Read the model definition and answer for the solid it produces. Units are mm, in the model's axes. A direction names the side the tool comes from. Coordinates: 2 decimals unless noted, no trailing zeros. Order: outer loops, then holes, each group sorted by start corner. A loop starts at its lowest first (then second) coordinate and runs counter-clockwise, first axis right, second up. Notation, with made-up numbers: M 6,49 L 59,49 A9 ccw 59,59 Z; hole C 63,57 d3. An arc over 180 degrees is marked long. Put each result on its own line as item: value.
from build123d import *

# Parameters (mm, degrees)
F0_R     = 1.5
F0_R_2   = 11
F1_DEPTH = 15
F2_W     = 10
F2_H     = 10
F3_DEPTH = 20
F4_W     = 15
F4_H     = 15
F4_W_2   = 10
F4_H_2   = 10
F5_DEPTH = 20
F6_F1_R  = 5
F6_F2_R  = 5
F6_F3_R  = 5
F6_F4_R  = 5
F6_F5_R  = 5
F6_F6_R  = 5
F6_F7_R  = 5
F6_F8_R  = 5
F6_F9_R  = 5
F6_F10_R = 5
F6_F11_R = 5
F6_F12_R = 5
F6_F13_R = 5
F7_R     = 4
F8_DEPTH = 7.5
F9_R     = 5


with BuildPart() as f1:
    # F0 (on Top) → F1 (new body)
    with BuildSketch(Plane.XY):
        with BuildLine():
            Line((-45, -32.5), (-45, -45))
            Line((-45, -45), (-30, -45))
            Line((-30, -45), (-30, -60))
            Line((-30, -60), (-15, -60))
            Line((-15, -60), (-15, -45))
            Line((-15, -45), (0, -45))
            Line((0, -45), (0, -32.5))
            ThreePointArc((0, -32.5), (10, -22.5), (0, -12.5))
            Line((0, -12.5), (0, 0))
            Line((0, 0), (-15, 0))
            Line((-15, 0), (-15, 15))
            Line((-15, 15), (-30, 15))
            Line((-30, 15), (-30, 0))
            Line((-30, 0), (-45, 0))
            Line((-45, 0), (-45, -12.5))
            ThreePointArc((-45, -12.5), (-55, -22.5), (-45, -32.5))
        make_face()
        with Locations((-38, -38)):
            Circle(F0_R, mode=Mode.SUBTRACT)
        with Locations((-7, -38)):
            Circle(F0_R, mode=Mode.SUBTRACT)
        with Locations((-38, -7)):
            Circle(F0_R, mode=Mode.SUBTRACT)
        with Locations((-22.5, -22.5)):
            Circle(F0_R_2, mode=Mode.SUBTRACT)
        with Locations((-7, -7)):
            Circle(F0_R, mode=Mode.SUBTRACT)
    extrude(amount=F1_DEPTH)

    # F2 (on face) → F3 (cut)
    with BuildSketch(Plane.XZ.offset(60)):
        with Locations((-22.5, 7.5)):
            Rectangle(F2_W, F2_H)
    extrude(amount=-F3_DEPTH, mode=Mode.SUBTRACT)

    # F4 (on face) → F5 (join)
    with BuildSketch(Plane.XY.offset(15)):
        with Locations((-22.5, 7.5)):
            Rectangle(F4_W, F4_H)
        with Locations((-22.5, 7.5)):
            Rectangle(F4_W_2, F4_H_2, mode=Mode.SUBTRACT)
    extrude(amount=F5_DEPTH)

    # F6: fillet of radius 5 on 13 edges, made by hand

    # F6_f1
    f6_f1_edges = [f1.edges().sort_by_distance(p)[0] for p in [
        (-15, 0, 7.5),
    ]]
    fillet(f6_f1_edges, radius=F6_F1_R)

    # F6_f2
    f6_f2_edges = [f1.edges().sort_by_distance(p)[0] for p in [
        (-22.5, 0, 15),
    ]]
    fillet(f6_f2_edges, radius=F6_F2_R)

    # F6_f3
    f6_f3_edges = [f1.edges().sort_by_distance(p)[0] for p in [
        (0, -12.5, 7.5),
    ]]
    fillet(f6_f3_edges, radius=F6_F3_R)

    # F6_f4
    f6_f4_edges = [f1.edges().sort_by_distance(p)[0] for p in [
        (0, 0, 7.5),
    ]]
    fillet(f6_f4_edges, radius=F6_F4_R)

    # F6_f5
    f6_f5_edges = [f1.edges().sort_by_distance(p)[0] for p in [
        (0, -32.5, 7.5),
    ]]
    fillet(f6_f5_edges, radius=F6_F5_R)

    # F6_f6
    f6_f6_edges = [f1.edges().sort_by_distance(p)[0] for p in [
        (0, -45, 7.5),
    ]]
    fillet(f6_f6_edges, radius=F6_F6_R)

    # F6_f7
    f6_f7_edges = [f1.edges().sort_by_distance(p)[0] for p in [
        (-15, -45, 7.5),
    ]]
    fillet(f6_f7_edges, radius=F6_F7_R)

    # F6_f8
    f6_f8_edges = [f1.edges().sort_by_distance(p)[0] for p in [
        (-30, -45, 7.5),
    ]]
    fillet(f6_f8_edges, radius=F6_F8_R)

    # F6_f9
    f6_f9_edges = [f1.edges().sort_by_distance(p)[0] for p in [
        (-45, -45, 7.5),
    ]]
    fillet(f6_f9_edges, radius=F6_F9_R)

    # F6_f10
    f6_f10_edges = [f1.edges().sort_by_distance(p)[0] for p in [
        (-45, -32.5, 7.5),
    ]]
    fillet(f6_f10_edges, radius=F6_F10_R)

    # F6_f11
    f6_f11_edges = [f1.edges().sort_by_distance(p)[0] for p in [
        (-45, -12.5, 7.5),
    ]]
    fillet(f6_f11_edges, radius=F6_F11_R)

    # F6_f12
    f6_f12_edges = [f1.edges().sort_by_distance(p)[0] for p in [
        (-45, 0, 7.5),
    ]]
    fillet(f6_f12_edges, radius=F6_F12_R)

    # F6_f13
    f6_f13_edges = [f1.edges().sort_by_distance(p)[0] for p in [
        (-30, 0, 7.5),
    ]]
    fillet(f6_f13_edges, radius=F6_F13_R)

    # F7 (on face) → F8 (cut)
    with BuildSketch(Plane.XY.offset(15)):
        with Locations((-45, -22.5)):
            Circle(F7_R)
        with Locations((0, -22.5)):
            Circle(F7_R)
    extrude(amount=-F8_DEPTH, mode=Mode.SUBTRACT)

    # F9
    f9_edges = [f1.edges().sort_by_distance(p)[0] for p in [
        (-15, 0, 15),
        (-30, 0, 15),
    ]]
    fillet(f9_edges, radius=F9_R)


solid = f1.part
Q1. Consider line 1 along Y through (x, z) = (-38, 11); line 2 along Y through (x, z) = (-22.5, 25.5); line 3 along Y through (x, z) = (-22.5, 11.75). Determine where each line is inside the solid, lowest interval first.
Answers below:
line 1: y = -45 to -39.5, -36.5 to -8.5, -5.5 to 0
line 2: y = 0 to 2.5, 12.5 to 15
line 3: y = -40 to -33.5, -11.5 to 15
Q2. Find section A-A on x = -38. Write down the section's boundary in (y, z).
Answers below:
outline: M -45,0 L -39.5,0 L -39.5,15 L -45,15 Z; M -36.5,0 L -8.5,0 L -8.5,15 L -36.5,15 Z; M -5.5,0 L 0,0 L 0,15 L -5.5,15 Z
Q3. Given pin 1 (1.7 mm diameter, centred on y = -38.5, z = 6.5, fed in from +X); pin 2 (5 mm diameter, centred on y = 7.5, z = 21.5, fed in from -X); pin 3 (5 mm diameter, centred on x = -45, y = -22.5, fed in from +Z), each flat-ended and moving along its own axis, determine where each tip first touches the part or whether it passes through.
Answers below:
pin 1: stops at x = 0
pin 2: stops at x = -30
pin 3: stops at z = 7.5
Q4. For a pull along Y with two mould halves and no side action, classify faces 1 (the face through (-45.943, -11.28, 7.605)), 2 (the face through (-45, -38, 7)), 3 (the face through (-17.5, 7, 25)) as +Y half, -Y half, draft (parallel to the pull), parting line (faces both ways), or undercut.
Answers below:
face 1: +Y half
face 2: draft
face 3: undercut
Q5. Find section C-C on z = 23.5. Write down the section's boundary in (x, y).
Answers below:
outline: M -30,0 L -15,0 L -15,15 L -30,15 Z; hole M -27.5,2.5 L -17.5,2.5 L -17.5,12.5 L -27.5,12.5 Z
Q6. A tool of negligible diameter and unlimited length cuts with its end or side. For faces 4 (the face through (0, -7, 7)), 5 (the face through (-23, 2.5, 25)), 6 (the face through (-15, -55, 7)), from which of +Z, -Z, +X, -X, +Y, -Y can it reach the whole face along a straight path? Write none if from no direction.
Answers below:
face 4: +Z, -Z, +X, +Y
face 5: +Z
face 6: +Z, -Z, +X, -Y
Q7. Find section B-B on y = -44. Write down the section's boundary in (x, z), plus the area to 3 significant figures.
Answers below:
outline: M -43,0 L -2,0 L -2,15 L -43,15 Z; hole M -27.5,2.5 L -17.5,2.5 L -17.5,12.5 L -27.5,12.5 Z
area: 515 mm^2
